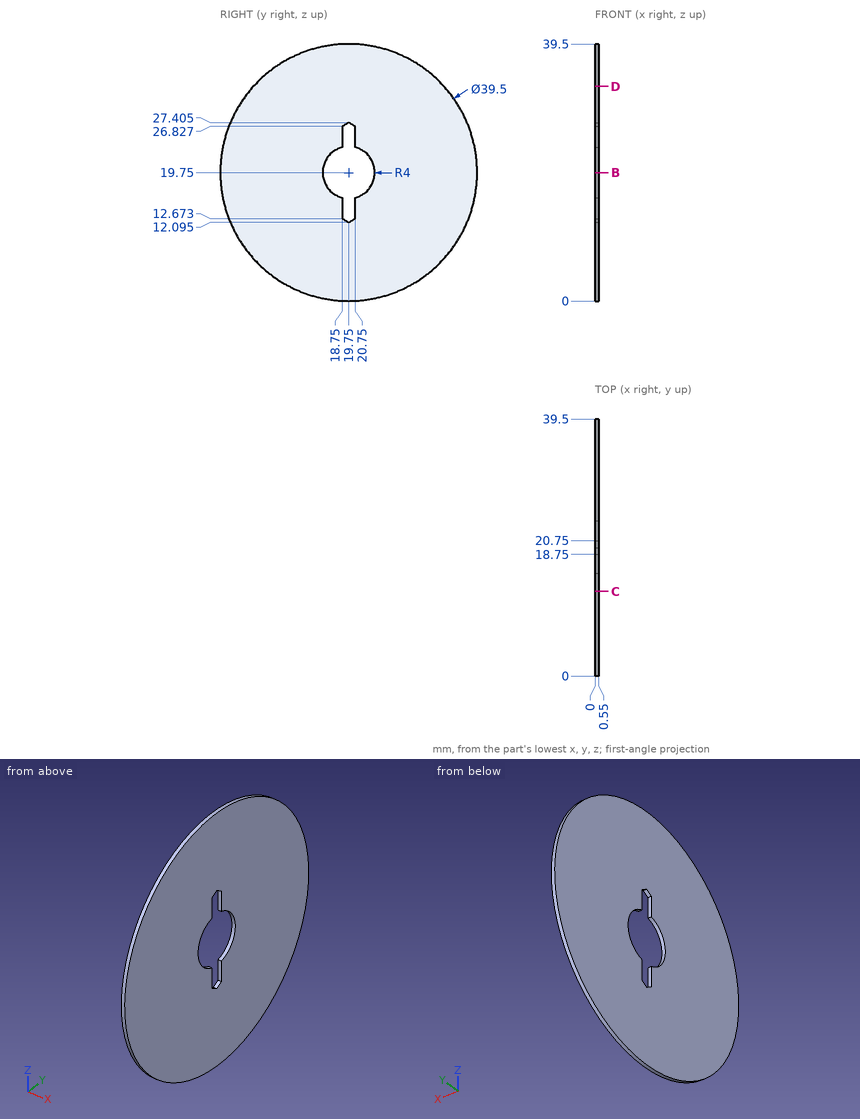
Here's the drawing with two shaded views (mm, measured from the low corner). I have some questions. Give positions to 0.01 mm unless a question says otherwise; leave off trailing zeros. Order: outer loops, then holes, each group sorted by start corner. A loop starts at its lowest first (then second) coordinate and runs counter-clockwise, first axis right, second up. Notation, with made-up numbers: M 71.5,24 L 101.5,24 A7 ccw 101.5,36 Z; hole C -24.5,-15 d8. An arc over 180 degrees is marked long. One line per item, written item: value.
1) I want a section at D-D, the plane z = 33. List the corners of the cut face in (x, y) for me.
Answer sheet:
outline: M 0,5.1 L 0.55,5.1 L 0.55,34.4 L 0,34.4 Z
2) Please list where these lines run through material, in increasing order: line 1 along Y through (x, z) = (0.3, 19.5); line 2 along Y through (x, z) = (0.4, 22).
Answer sheet:
line 1: y = 0 to 15.76, 23.74 to 39.5
line 2: y = 0.13 to 16.44, 23.06 to 39.37
3) I want a section at B-B, the plane z = 19.75. List the corners of the cut face in (x, y) for me.
Answer sheet:
outline: M 0,0 L 0.55,0 L 0.55,15.75 L 0,15.75 Z; M 0,23.75 L 0.55,23.75 L 0.55,39.5 L 0,39.5 Z
4) I want a section at C-C, the plane y = 13. List the corners of the cut face in (x, z) for me.
Answer sheet:
outline: M 0,1.19 L 0.55,1.19 L 0.55,38.31 L 0,38.31 Z
